```python
from build123d import *

# Parameters (mm, degrees)
BOSS_EXTRUDE1_DEPTH = 1.5
SKETCH17_W          = 59.095547363
SKETCH17_H          = 97.719033267
CUT_EXTRUDE2_DEPTH  = 165.658179571


with BuildPart() as part:
    # Sketch1 → Boss-Extrude1 (new body)
    with BuildSketch(Plane(origin=(0, 0, 0), x_dir=(-1, 0, 0), z_dir=(0, -1, 0))):
        with BuildLine():
            Line((-68.228994051, -80.900990016), (-68.228994051, 14.099009984))
            add(Edge.make_bspline(
                [(-61.728994051, 35.999084059), (-62.421478219, 17.933639863), (-67.544211434, 25.081077147), (-68.540266051, 21.159243181), (-68.228994051, 14.099009984)],
                knots=[0, 0, 0, 0, 0, 1, 1, 1, 1, 1], degree=4))
            Line((-61.728994051, 35.999084059), (-61.728994051, 115.999084059))
            add(Edge.make_bspline(
                [(-61.728994051, 115.999084059), (-61.589708219, 128.711907965), (-56.064830782, 140.140701438), (-48.600220127, 149.828937742)],
                knots=[0, 0, 0, 0, 1, 1, 1, 1], degree=3))
            Line((-48.600220127, 149.828937742), (-24.857767976, 149.828937742))
            add(Edge.make_bspline(
                [(-11.728994051, 115.999084059), (-11.868279883, 128.711907965), (-17.39315732, 140.140701438), (-24.857767976, 149.828937742)],
                knots=[0, 0, 0, 0, 1, 1, 1, 1], degree=3))
            Line((-11.728994051, 115.999084059), (-11.728994051, 35.999084059))
            add(Edge.make_bspline(
                [(-11.728994051, 35.999084059), (-11.036509883, 17.933639863), (-5.913776668, 25.081077147), (-4.917722051, 21.159243181), (-5.228994051, 14.099009984)],
                knots=[0, 0, 0, 0, 0, 1, 1, 1, 1, 1], degree=4))
            Line((-5.228994051, 14.099009984), (-5.228994051, -80.900990016))
            Line((-5.228994051, -80.900990016), (-68.228994051, -80.900990016))
        make_face()
    extrude(amount=BOSS_EXTRUDE1_DEPTH)

    # Sketch17 → Cut-Extrude2 (cut, through all)
    with BuildSketch(Plane(origin=(0, 0, 0), x_dir=(1, 0, 0), z_dir=(0, 1, 0))):
        with Locations((36.634404956, -29.217068725)):
            Rectangle(SKETCH17_W, SKETCH17_H)
    extrude(amount=-CUT_EXTRUDE2_DEPTH, mode=Mode.SUBTRACT)


solid = part.part
```
Check sheet for the modelled part. Datum: model origin and axes. Units: mm. Round coordinates to 2 decimals unless told otherwise and drop trailing zeros. Write each loop counter-clockwise with the first axis right and the second up, starting at its lowest first coordinate (ties: lowest second). Pieces come first, ordered by that corner, then holes. Notation, with made-up numbers: (85, 89.5) -> (92, 89.5) arc R29 ccw to (92, 128.5) -> close; hole circle Ø11 at (38.5, 8). An arc over 180 degrees is marked (long way). One line per question, with ' | ' between items. Start each with the question number.
1. Depth check by flat-ended pin: pin 1 (0.8 mm diameter, centred on y = -1, z = -80.5, fed in from +X); pin 2 (0.8 mm diameter, centred on y = -1, z = 8.5, fed in from -X). Enter the tip coordinate at first touch or a pass-through.
2. Sectioned sample at C-C, the plane z = -75. Record the cut outline in (x, y), then the cut area to 3 significant figures.
3. Scan lines: line 1 along Z through (x, y) = (34, -0.15); line 2 along X through (y, z) = (-0.65, 29); line 3 along X through (y, z) = (-0.1, -82). Record each from-to range of solid material in increasing order. Write a range as from..to.
4. Sectioned sample at A-A, the plane x = 46. Record the cut outline in (y, z), then the cut area to 3 significant figures.
5. Sectioned sample at B-B, the plane z = 59. Record the cut outline in (x, y).
Taken from the geometry:
1) pin 1: stops at x = 61.73 | pin 2: stops at x = 5.23
2) outline: (11.73, -1.5) -> (61.73, -1.5) -> (61.73, 0) -> (11.73, 0) -> close | area: 75.0 mm^2
3) line 1: z = -149.83..-19.64, 78.08..80.9 | line 2: x = 5.23..7.09, 66.18..68.23 | line 3: x = 11.73..61.73
4) outline: (-1.5, -149.83) -> (0, -149.83) -> (0, -19.64) -> (-1.5, -19.64) -> close; (-1.5, 78.08) -> (0, 78.08) -> (0, 80.9) -> (-1.5, 80.9) -> close | area: 200 mm^2
5) outline: (5.23, -1.5) -> (7.09, -1.5) -> (7.09, 0) -> (5.23, 0) -> close; (66.18, -1.5) -> (68.23, -1.5) -> (68.23, 0) -> (66.18, 0) -> close
